Design review of the part built by this model. Coordinates are the model's own, in mm. Face numbers are marked on the shaded views. A direction names the side the tool comes from. Coordinates: 2 decimals unless noted, no trailing zeros. Write each loop counter-clockwise with the first axis right and the second up, starting at its lowest first coordinate (ties: lowest second). Pieces come first, ordered by that corner, then holes.
Q1. The part is to be moulded in two halves that separate along X. For the marked faces 5 and 6, say which applies: +X half, -X half, draft (parallel to the pull), parting line (faces both ways), or undercut.
Q2. Add section C-C, the plane y = 18. Give the boundary of the cut face in (x, z).
Q3. Clearance check with flat-ended pins moving along their axes: pin 1 Ø3 at (y, z) = (24, -12) entering from +X; pin 2 Ø3 at (y, z) = (7, -30) entering from -X; pin 3 Ø3 at (y, z) = (21, -23) entering from +X; pin 4 Ø1.5 at (y, z) = (26, -28.5) entering from +X. State where each tip first meets the part, or that it passes through.
Q4. Machinability: for the marked faces 1, 2, 3 and 4, which of the approach directions +Z, -Z, +X, -X, +Y, -Y give a long, thin tool a straight path to every point of the face, cutting with its end or side? Answer none if there is none.
Q5. Add section A-A, the plane x = 0. Give the number of separate pieces and of enclosed holes in the cut face, plus the area to 3 significant figures.
Q6. Add section B-B, the plane y = 13.5. Give the boundary of the cut face in (x, z), plus the area to 3 significant figures.
Q7. To check wall thickness, follow probe 1 along X at (y, z) = (27, 0); probe 2 along Z at (x, y) = (0, 8); probe 3 along X at (y, z) = (1.1, -42.5). State the ranges of each line that lie inside material, in increasing order.
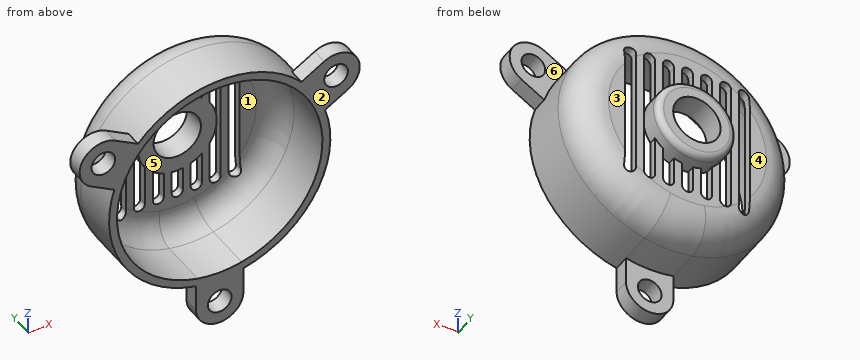
from build123d import *

# Parameters (mm, degrees)
BOSS_EXTRUDE1_DEPTH = 25
FILLET1_R           = 10
SHELL1_T            = -2.5
SKETCH1_3_R         = 3.75
BOSS_EXTRUDE2_DEPTH = 5
CUT_EXTRUDE1_DEPTH  = 35
SKETCH4_R           = 12.5
SKETCH4_R_2         = 7.5
BOSS_EXTRUDE3_DEPTH = 7.5
SKETCH4_3_R         = 7.5
CUT_EXTRUDE2_DEPTH  = 18.75
FILLET2_R           = 2


with BuildPart() as part:
    # Sketch1 → Boss-Extrude1 (new body)
    with BuildSketch(Plane(origin=(0, 0, 0), x_dir=(1, 0, 0), z_dir=(0, 1, 0))):
        with BuildLine():
            ThreePointArc((-7.5, 34.186985828), (0, 35), (7.5, 34.186985828))
            ThreePointArc((7.5, 34.186985828), (0, -35), (-7.5, 34.186985828))
        make_face()
    extrude(amount=BOSS_EXTRUDE1_DEPTH)

    # Fillet1
    fillet1_edges = [part.edges().sort_by_distance(p)[0] for p in [
        (7.5, 25, 34.186985828),
    ]]
    fillet(fillet1_edges, radius=FILLET1_R)

    # Shell1
    shell1_openings = [part.faces().sort_by_distance(p)[0] for p in [
        (0, 0, 0),
    ]]
    offset(amount=SHELL1_T, openings=shell1_openings, kind=Kind.INTERSECTION)

    # Sketch1_3 → Boss-Extrude2 (add)
    # profile 1 of 3: a face of its own
    with BuildSketch(Plane(origin=(0, 0, 0), x_dir=(1, 0, 0), z_dir=(0, 1, 0))):
        with BuildLine():
            Line((40.556079661, -14.754809472), (33.356798206, -10.598302386))
            ThreePointArc((33.356798206, -10.598302386), (30.310889132, -17.5), (25.856798206, -23.588683442))
            Line((25.856798206, -23.588683442), (33.056079661, -27.745190528))
            ThreePointArc((33.056079661, -27.745190528), (43.301270189, -25), (40.556079661, -14.754809472))
        make_face()
        with Locations(Location((36.806079661, -21.25, 0), (0, 0, 270))):
            Circle(SKETCH1_3_R, mode=Mode.SUBTRACT)
    # profile 2 of 3: a face of its own
    with BuildSketch(Plane(origin=(0, 0, 0), x_dir=(1, 0, 0), z_dir=(0, 1, 0))):
        with BuildLine():
            ThreePointArc((-25.856798206, -23.588683442), (-30.310889132, -17.5), (-33.356798206, -10.598302386))
            Line((-33.356798206, -10.598302386), (-40.556079661, -14.754809472))
            ThreePointArc((-40.556079661, -14.754809472), (-43.301270189, -25), (-33.056079661, -27.745190528))
            Line((-33.056079661, -27.745190528), (-25.856798206, -23.588683442))
        make_face()
        with Locations(Location((-36.806079661, -21.25, 0), (0, 0, 270))):
            Circle(SKETCH1_3_R, mode=Mode.SUBTRACT)
    # profile 3 of 3: a face of its own
    with BuildSketch(Plane(origin=(0, 0, 0), x_dir=(1, 0, 0), z_dir=(0, 1, 0))):
        with BuildLine():
            Line((-7.5, 42.5), (-7.5, 34.186985828))
            ThreePointArc((-7.5, 34.186985828), (0, 35), (7.5, 34.186985828))
            Line((7.5, 34.186985828), (7.5, 42.5))
            ThreePointArc((7.5, 42.5), (0, 50), (-7.5, 42.5))
        make_face()
        with Locations(Location((0, 42.5, 0), (0, 0, 270))):
            Circle(SKETCH1_3_R, mode=Mode.SUBTRACT)
    extrude(amount=BOSS_EXTRUDE2_DEPTH)

    # Sketch2 → Cut-Extrude1 (cut)
    with BuildSketch(Plane.XZ):
        with BuildLine():
            Line((-10.25, 20), (-10.25, -20))
            ThreePointArc((-10.25, -20), (-12, -21.75), (-13.75, -20))
            Line((-13.75, -20), (-13.75, 20))
            ThreePointArc((-13.75, 20), (-12, 21.75), (-10.25, 20))
        make_face()
        with BuildLine():
            Line((-19.75, 20), (-19.75, -20))
            ThreePointArc((-19.75, -20), (-18, -21.75), (-16.25, -20))
            Line((-16.25, -20), (-16.25, 20))
            ThreePointArc((-16.25, 20), (-18, 21.75), (-19.75, 20))
        make_face()
        with BuildLine():
            Line((-4.25, 20), (-4.25, -20))
            ThreePointArc((-4.25, -20), (-6, -21.75), (-7.75, -20))
            Line((-7.75, -20), (-7.75, 20))
            ThreePointArc((-7.75, 20), (-6, 21.75), (-4.25, 20))
        make_face()
        with BuildLine():
            Line((1.75, 20), (1.75, -20))
            ThreePointArc((1.75, -20), (0, -21.75), (-1.75, -20))
            Line((-1.75, -20), (-1.75, 20))
            ThreePointArc((-1.75, 20), (0, 21.75), (1.75, 20))
        make_face()
        with BuildLine():
            Line((7.75, 20), (7.75, -20))
            ThreePointArc((7.75, -20), (6, -21.75), (4.25, -20))
            Line((4.25, -20), (4.25, 20))
            ThreePointArc((4.25, 20), (6, 21.75), (7.75, 20))
        make_face()
        with BuildLine():
            Line((13.75, 20), (13.75, -20))
            ThreePointArc((13.75, -20), (12, -21.75), (10.25, -20))
            Line((10.25, -20), (10.25, 20))
            ThreePointArc((10.25, 20), (12, 21.75), (13.75, 20))
        make_face()
        with BuildLine():
            Line((19.75, 20), (19.75, -20))
            ThreePointArc((19.75, -20), (18, -21.75), (16.25, -20))
            Line((16.25, -20), (16.25, 20))
            ThreePointArc((16.25, 20), (18, 21.75), (19.75, 20))
        make_face()
    extrude(amount=-CUT_EXTRUDE1_DEPTH, mode=Mode.SUBTRACT)

    # Sketch4 → Boss-Extrude3 (add)
    # profile 1 of 2: a face of its own
    with BuildSketch(Plane.XZ.offset(-22.5)):
        with Locations(Location((0, 0, 0), (0, 0, 270))):
            Circle(SKETCH4_R)
        Circle(SKETCH4_R_2, mode=Mode.SUBTRACT)
    # profile 2 of 2: a face of its own
    with BuildSketch(Plane.XZ.offset(-22.5)):
        Circle(SKETCH4_R_2)
    extrude(amount=-BOSS_EXTRUDE3_DEPTH)

    # Sketch4_3 → Cut-Extrude2 (cut, symmetric)
    with BuildSketch(Plane.XZ.offset(-22.5)):
        with Locations(Location((0, 0, 0), (0, 0, 270))):
            Circle(SKETCH4_3_R)
    extrude(amount=CUT_EXTRUDE2_DEPTH, both=True, mode=Mode.SUBTRACT)

    # Fillet2
    fillet2_edges = [part.edges().sort_by_distance(p)[0] for p in [
        (0, 30, 12.5),
    ]]
    fillet(fillet2_edges, radius=FILLET2_R)


solid = part.part
Here are the results:
1. face 5: undercut
1. face 6: draft
2. outline: circle Ø69.08 at (0, 0); hole circle Ø63.75 at (0, 0)
3. pin 1: stops at x = 29.34
3. pin 2: stops at x = -20.32
3. pin 3: stops at x = 25.58
3. pin 4: passes through
4. face 1: -Y
4. face 2: +Z, -Z, +X, -X, -Y
4. face 3: +Z, -Z, +X, +Y
4. face 4: +Z, -Z, -X, +Y
5. separate pieces: 5
5. enclosed holes: 0
5. area: 271 mm2
6. outline: circle Ø70 at (0, 0); hole circle Ø65 at (0, 0)
6. area: 530 mm2
7. probe 1: x = -12.5 to -7.5, 7.5 to 12.5
7. probe 2: z = -35 to -32.5, 32.5 to 35
7. probe 3: x = -7.5 to -3.75, 3.75 to 7.5
